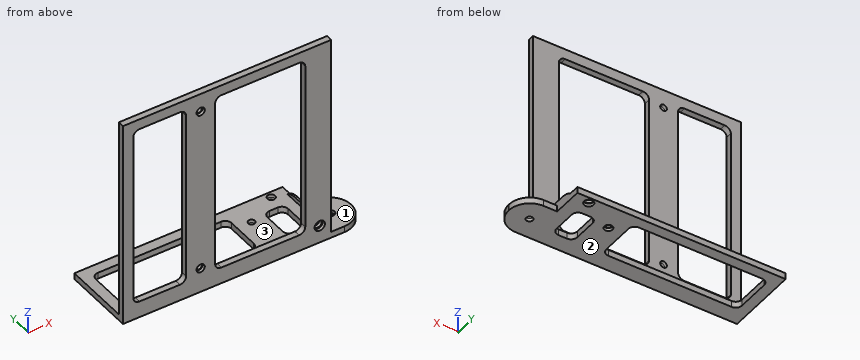
from build123d import *

# Parameters (mm, degrees)
SKETCH1_R           = 1.6
SKETCH1_R_2         = 1.875
BOSS_EXTRUDE1_DEPTH = 3
BOSS_EXTRUDE2_DEPTH = 101
SKETCH1_5_W         = 1
SKETCH1_5_H         = 27
BOSS_EXTRUDE3_DEPTH = 5
SKETCH2_W           = 16.5
SKETCH2_H           = 14.6
CUT_EXTRUDE1_DEPTH  = 5
SKETCH3_W           = 16.5
SKETCH3_H           = 98
CUT_EXTRUDE2_DEPTH  = 5
FILLET1_R           = 10
FILLET2_R           = 10
SKETCH4_R           = 1.6
SKETCH4_R_2         = 1.875
CUT_EXTRUDE3_DEPTH  = 5
FILLET3_R           = 10
SKETCH5_R           = 2
SKETCH5_R_2         = 2.5
CUT_EXTRUDE4_DEPTH  = 1.5
SKETCH6_R           = 2
CUT_EXTRUDE5_DEPTH  = 1.5
SKETCH7_R           = 2
SKETCH7_R_2         = 2.25
CUT_EXTRUDE6_DEPTH  = 1.5
SKETCH8_W           = 25.5
SKETCH8_H           = 88
SKETCH8_W_2         = 43.5
CUT_EXTRUDE7_DEPTH  = 10
FILLET4_R           = 3
SKETCH9_W           = 65.5
SKETCH9_H           = 22
SKETCH9_W_2         = 10
SKETCH9_H_2         = 17
CUT_EXTRUDE8_DEPTH  = 10
FILLET5_R           = 3


with BuildPart() as part:
    # Sketch1 → Boss-Extrude1 (new body)
    # profile 1 of 2: a face of its own
    with BuildSketch(Plane.XY):
        Polygon((0, 3), (0, 0), (117, 0), (117, 3), (100.5, 3), (99.5, 3), align=None)
    # profile 2 of 2: a face of its own
    with BuildSketch(Plane.XY):
        Polygon((0, 35), (0, 3), (99.5, 3), (99.5, 30), (100.5, 30), (100.5, 3), (117, 3), (117, 35), align=None)
        with Locations((107, 10.2)):
            Circle(SKETCH1_R, mode=Mode.SUBTRACT)
        with Locations((77.5, 23)):
            Circle(SKETCH1_R, mode=Mode.SUBTRACT)
        with Locations((93, 32)):
            Circle(SKETCH1_R_2, mode=Mode.SUBTRACT)
    extrude(amount=BOSS_EXTRUDE1_DEPTH)

    # Sketch1<4> → Boss-Extrude2 (add)
    with BuildSketch(Plane.XY):
        Polygon((0, 3), (0, 0), (117, 0), (117, 3), (100.5, 3), (99.5, 3), align=None)
    extrude(amount=BOSS_EXTRUDE2_DEPTH)

    # Sketch1<5> → Boss-Extrude3 (add)
    with BuildSketch(Plane.XY):
        with Locations((100, 16.5)):
            Rectangle(SKETCH1_5_W, SKETCH1_5_H)
    extrude(amount=BOSS_EXTRUDE3_DEPTH)

    # Sketch2 → Cut-Extrude1 (cut)
    with BuildSketch(Plane.XY.offset(3)):
        with Locations((108.75, 27.7)):
            Rectangle(SKETCH2_W, SKETCH2_H)
    extrude(amount=-CUT_EXTRUDE1_DEPTH, mode=Mode.SUBTRACT)

    # Sketch3 → Cut-Extrude2 (cut)
    with BuildSketch(Plane(origin=(0, 3, 0), x_dir=(1, 0, 0), z_dir=(0, 1, 0))):
        with Locations((108.75, -52)):
            Rectangle(SKETCH3_W, SKETCH3_H)
    extrude(amount=-CUT_EXTRUDE2_DEPTH, mode=Mode.SUBTRACT)

    # Fillet1
    fillet1_edges = [part.edges().sort_by_distance(p)[0] for p in [
        (117, 20.4, 1.5),
    ]]
    fillet(fillet1_edges, radius=FILLET1_R)

    # Fillet2
    fillet2_edges = [part.edges().sort_by_distance(p)[0] for p in [
        (117, 0, 1.5),
    ]]
    fillet(fillet2_edges, radius=FILLET2_R)

    # Sketch4 → Cut-Extrude3 (cut)
    with BuildSketch(Plane(origin=(0, 3, 0), x_dir=(1, 0, 0), z_dir=(0, 1, 0))):
        with Locations(Location((37.5, -12, 0), (0, 0, 270))):
            Circle(SKETCH4_R)
        with Locations(Location((37.5, -92, 0), (0, 0, 270))):
            Circle(SKETCH4_R)
        with Locations(Location((95, -8.5, 0), (0, 0, 270))):
            Circle(SKETCH4_R_2)
    extrude(amount=-CUT_EXTRUDE3_DEPTH, mode=Mode.SUBTRACT)

    # Fillet3
    # the kernel refuses this fillet: 10 mm, written as the material it takes off along each edge
    with BuildSketch(Plane(origin=(84.5, 30, 5), x_dir=(0, 0, -1), z_dir=(1, 0, 0))) as fillet3_piece_1:
        with BuildLine():
            CenterArc((10, -6), FILLET3_R, 143.130102354, 36.869897646)
            Line((0, -6), (-0.2, -6))
            Line((-0.2, -6), (-0.2, 0))
            Line((-0.2, 0), (0, 0.2))
            ThreePointArc((0, 0.2), (1, 0.2), (1.84, 0.12))
            Line((1.84, 0.12), (2, 0))
        make_face()
    extrude(amount=31, mode=Mode.SUBTRACT)

    # Sketch5 → Cut-Extrude4 (cut)
    with BuildSketch(Plane.XZ):
        with Locations(Location((37.5, 92, 0), (0, 0, 270))):
            Circle(SKETCH5_R)
        with Locations(Location((37.5, 12, 0), (0, 0, 270))):
            Circle(SKETCH5_R)
        with Locations(Location((95, 8.5, 0), (0, 0, 270))):
            Circle(SKETCH5_R_2)
    extrude(amount=-CUT_EXTRUDE4_DEPTH, mode=Mode.SUBTRACT)

    # Sketch6 → Cut-Extrude5 (cut)
    with BuildSketch(Plane.XY.offset(3)):
        with Locations((107, 10.2)):
            Circle(SKETCH6_R)
    extrude(amount=-CUT_EXTRUDE5_DEPTH, mode=Mode.SUBTRACT)

    # Sketch7 → Cut-Extrude6 (cut)
    with BuildSketch(Plane(origin=(0, 0, 0), x_dir=(-1, 0, 0), z_dir=(0, 0, -1))):
        with Locations((-77.5, 23)):
            Circle(SKETCH7_R)
        with Locations((-93, 32)):
            Circle(SKETCH7_R_2)
    extrude(amount=-CUT_EXTRUDE6_DEPTH, mode=Mode.SUBTRACT)

    # Sketch8 → Cut-Extrude7 (cut)
    with BuildSketch(Plane(origin=(0, 3, 0), x_dir=(1, 0, 0), z_dir=(0, 1, 0))):
        with Locations((17.75, -52)):
            Rectangle(SKETCH8_W, SKETCH8_H)
        with Locations((66.25, -52)):
            Rectangle(SKETCH8_W_2, SKETCH8_H)
    extrude(amount=-CUT_EXTRUDE7_DEPTH, mode=Mode.SUBTRACT)

    # Fillet4
    fillet4_edges = [part.edges().sort_by_distance(p)[0] for p in [
        (5, 1.5, 96),
        (5, 1.5, 8),
        (30.5, 1.5, 8),
        (30.5, 1.5, 96),
        (44.5, 1.5, 96),
        (44.5, 1.5, 8),
        (88, 1.5, 8),
        (88, 1.5, 96),
    ]]
    fillet(fillet4_edges, radius=FILLET4_R)

    # Sketch9 → Cut-Extrude8 (cut)
    with BuildSketch(Plane.XY.offset(3)):
        with Locations((37.75, 19)):
            Rectangle(SKETCH9_W, SKETCH9_H)
        with Locations((89.5, 16.5)):
            Rectangle(SKETCH9_W_2, SKETCH9_H_2)
    extrude(amount=-CUT_EXTRUDE8_DEPTH, mode=Mode.SUBTRACT)

    # Fillet5
    fillet5_edges = [part.edges().sort_by_distance(p)[0] for p in [
        (5, 8, 1.5),
        (5, 30, 1.5),
        (70.5, 30, 1.5),
        (70.5, 8, 1.5),
        (84.5, 8, 1.5),
        (84.5, 25, 1.5),
        (94.5, 25, 1.5),
        (94.5, 8, 1.5),
    ]]
    fillet(fillet5_edges, radius=FILLET5_R)


solid = part.part
CAD build for the part. Positions are in the model's coordinates, mm. Face numbers are marked on the shaded views. A direction names the side the tool comes from. Round coordinates to 2 decimals unless told otherwise and drop trailing zeros. Order: outer loops, then holes, each group sorted by start corner. A loop starts at its lowest first (then second) coordinate and runs counter-clockwise, first axis right, second up. Notation, with made-up numbers: (47.25, -11) -> (85.25, -11) arc R18 ccw to (85.25, 14) -> close; hole circle Ø6 at (-31.75, 76.25). An arc over 180 degrees is marked (long way). Write item = value, one per line. Start each with the question number.
(1) Which spindle directions (+Z, -Z, +X, -X, +Y, -Y) get a long thin tool onto all of the face, cutting with end or side? Do the marked faces 1, 2 and 3. Say none if no direction does.
(2) Probe line 1 (X direction, y = 2, z = 12); line 2 (X direction, y = 1, z = 92); line 3 (Z direction, x = 39, y = 31.5). List the from-to ranges inside material, lowest first. Write a range as [from, to].
(3) Cut at A-A, the plane z = 32. List the corners of the cut face in (x, y).
(4) Cut at C-C, the plane x = 32.5. List the corners of the cut face in (y, z), then the cut area to 3 significant figures.
(5) Pin check, flat tips, straight feed: P1, Ø5, axis at x = 112, y = 11, coming from the +Z side; P2, Ø12, axis at x = 83, z = 77.5, coming from the +Y side; P3, Ø2, axis at y = 19.5, z = 4.5, coming from the -X side. Stop position of each tip, or through.
(6) Cut at B-B, the plane x = 77.5. List the corners of the cut face in (y, z), then the cut area to 3 significant figures.
Model answer:
q1.face_1 = +Z, +X, +Y, -Y
q1.face_2 = -Z, +X, -X, +Y, -Y
q1.face_3 = +Z, -X, +Y
q2.line_1 = [0, 5], [30.5, 35.9], [39.1, 44.5], [88, 100.5]
q2.line_2 = [0, 5], [30.5, 35.5], [39.5, 44.5], [88, 100.5]
q2.line_3 = [0, 3]
q3.outline = (0, 0) -> (5, 0) -> (5, 3) -> (0, 3) -> close; (30.5, 0) -> (44.5, 0) -> (44.5, 3) -> (30.5, 3) -> close; (88, 0) -> (100.5, 0) -> (100.5, 3) -> (88, 3) -> close
q4.outline = (0, 0) -> (8, 0) -> (8, 3) -> (3, 3) -> (3, 101) -> (0, 101) -> close; (30, 0) -> (35, 0) -> (35, 3) -> (30, 3) -> close
q4.area = 333 mm2
q5.P1 = 3
q5.P2 = 3
q5.P3 = 99.5
q6.outline = (0, 0) -> (21, 0) -> (21, 1.5) -> (21.4, 1.5) -> (21.4, 3) -> (3, 3) -> (3, 8) -> (0, 8) -> close; (0, 96) -> (3, 96) -> (3, 101) -> (0, 101) -> close; (24.6, 1.5) -> (25, 1.5) -> (25, 0) -> (35, 0) -> (35, 3) -> (24.6, 3) -> close
q6.area = 124 mm2
